Design review of the part built by this model. Coordinates are the model's own, in mm. Face numbers are marked on the shaded views. Coordinates: 2 decimals unless noted, no trailing zeros. Order: outer loops, then holes, each group sorted by start corner. A loop starts at its lowest first (then second) coordinate and runs counter-clockwise, first axis right, second up. Notation, with made-up numbers: (44, 60.5) - (67, 60.5) arc R14 ccw to (67, 79.5) - close; hole circle Ø6 at (3.25, 0). An arc over 180 degrees is marked (long way). Write each question's results on one line, items separated by ' | '. Start each with the question number.
```python
from build123d import *

# Parameters (mm, degrees)
F1_DEPTH = 31.75


with BuildPart() as f1:
    # F0 (on Front) → F1 (new body)
    with BuildSketch(Plane.XZ):
        with BuildLine():
            Line((-41.549053, -55.585895), (41.549053, -55.585895))
            Line((41.549053, -55.585895), (41.549053, 55.585895))
            ThreePointArc((41.549053, 55.585895), (0, 97.134948), (-41.549053, 55.585895))
            Line((-41.549053, 55.585895), (-41.549053, -55.585895))
        make_face()
        with BuildLine():
            ThreePointArc((-23.30116, 55.585895), (0, 78.887055), (23.30116, 55.585895))
            ThreePointArc((23.30116, 55.585895), (0, 32.284735), (-23.30116, 55.585895))
        make_face(mode=Mode.SUBTRACT)
    extrude(amount=F1_DEPTH)


solid = f1.part
```
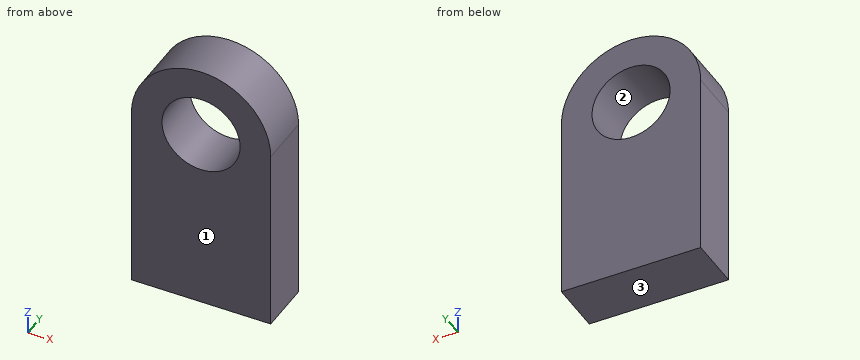
(1) Take a section at D-D (x = -33). State the section outline as (y, z) points, plus the area to 3 significant figures.
(2) Take a section at B-B (z = 44.5). State the section outline as (x, y) points.
(3) Mouldability with a two-part tool opening along Z and no side actions: class the marked faces 1, 2 and 3 as +Z half, -Z half, draft (parallel to the pull), parting line (faces both ways), or undercut.
(4) Take a section at A-A (x = 0). State the section outline as (y, z) points, plus the area to 3 significant figures.
(5) Take a section at C-C (y = -22.5). State the section outline as (x, z) points.
(6) Clearance check with a flat-ended pin moving along its axis: pin 1 (5 mm diameter, centred on x = 11.5, y = -18, fed in from +Z). State where the tip first meets the part, or that it passes through.
(7) To check wall thickness, follow line 1 along Z through (x, y) = (0, -16); line 2 along Z through (x, y) = (-17.5, -8); line 3 along Z through (x, y) = (-36, -25). State the ranges of each line that lie inside material, in increasing order. Write a range as [from, to].
Worked out:
1) outline: (-31.75, -55.59) - (0, -55.59) - (0, 80.83) - (-31.75, 80.83) - close | area: 4,330 mm^2
2) outline: (-41.55, -31.75) - (-20.5, -31.75) - (-20.5, 0) - (-41.55, 0) - close; (20.5, -31.75) - (41.55, -31.75) - (41.55, 0) - (20.5, 0) - close
3) face 1: draft | face 2: undercut | face 3: -Z half
4) outline: (-31.75, -55.59) - (0, -55.59) - (0, 32.28) - (-31.75, 32.28) - close; (-31.75, 78.89) - (0, 78.89) - (0, 97.13) - (-31.75, 97.13) - close | area: 3,370 mm^2
5) outline: (-41.55, -55.59) - (41.55, -55.59) - (41.55, 55.59) arc R41.55 ccw to (-41.55, 55.59) - close; hole circle Ø46.6 at (0, 55.59)
6) pin 1: z = 96.15
7) line 1: [-55.59, 32.28], [78.89, 97.13] | line 2: [-55.59, 40.2], [70.97, 93.27] | line 3: [-55.59, 76.33]
